Work out the finished part from the listing and answer in its coordinate system (mm). Face numbers are marked on the shaded views. A direction names the side the tool comes from. Give positions to 0.01 mm unless a question says otherwise; leave off trailing zeros. Order: outer loops, then holes, each group sorted by start corner. A loop starts at its lowest first (then second) coordinate and runs counter-clockwise, first axis right, second up. Notation, with made-up numbers: M -35.5,-1 L 10.5,-1 A31 cw 10.5,26 Z; hole C 17,-36.5 d9. An arc over 180 degrees is marked long. One line per item, written item: value.
from build123d import *

# Parameters (mm, degrees)
ESQUISSE1_R             = 24.5
BOSS_EXTRU_1_DEPTH      = 5
ESQUISSE2_R             = 25
BOSS_EXTRU_2_DEPTH      = 2
BOSS_EXTRU_4_START      = 2
ESQUISSE5_R             = 25
BOSS_EXTRU_4_DEPTH      = 2
ESQUISSE4_R             = 1.75
ENL_V_MAT_EXTRU_1_DEPTH = 37.482872694


with BuildPart() as part:
    # Esquisse1 → Boss.-Extru.1 (new body)
    with BuildSketch(Plane.XY):
        Circle(ESQUISSE1_R)
    extrude(amount=BOSS_EXTRU_1_DEPTH)

    # Esquisse2 → Boss.-Extru.2 (add)
    with BuildSketch(Plane(origin=(0, 0, 0), x_dir=(-1, 0, 0), z_dir=(0, 0, -1))):
        Circle(ESQUISSE2_R)
    extrude(amount=BOSS_EXTRU_2_DEPTH)

    # Esquisse5 → Boss.-Extru.4 (add)
    with BuildSketch(Plane.XY.offset(5).offset(BOSS_EXTRU_4_START)):
        with Locations(Location((0, 0, 0), (0, 0, 180))):
            Circle(ESQUISSE5_R)
    extrude(amount=-BOSS_EXTRU_4_DEPTH)

    # Esquisse4 → Enlèv. mat.-Extru.1 (cut, through all)
    with BuildSketch(Plane(origin=(0, 0, -2), x_dir=(-1, 0, 0), z_dir=(0, 0, -1))):
        Circle(ESQUISSE4_R)
    extrude(amount=-ENL_V_MAT_EXTRU_1_DEPTH, mode=Mode.SUBTRACT)


solid = part.part
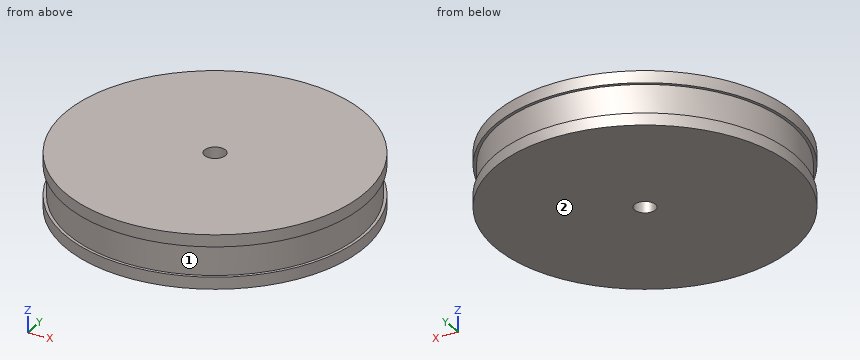
(1) Which of the six approach directions +Z, -Z, +X, -X, +Y, -Y give full straight-line access (tool end or side, diameter ignored) to the marked faces 1 and 2?
Findings:
face 1: none
face 2: -Z, +X, -X, +Y, -Y
(2) Section D-D, the plane y = 18.5 is taken. Give the vertices of the cut face in (x, z).
Findings:
outline: M -16.82,-2 L 16.82,-2 L 16.82,0 L 16.06,0 L 16.06,5 L 16.82,5 L 16.82,7 L -16.82,7 L -16.82,5 L -16.06,5 L -16.06,0 L -16.82,0 Z
(3) Section C-C, the plane z = 3.75 is taken. Give the vertices of the cut face in (x, y), then the cut area to 3 significant figures.
Findings:
outline: C 0,0 d49; hole C 0,0 d3.5
area: 1,880 mm^2
(4) Given P1, Ø3, axis at y = 9.5, z = 3, coming from the +X side; P2, Ø2, axis at y = -2.5, z = 2, coming from the +X side; P3, Ø2, axis at y = 1.5, z = -0.5, coming from the +X side (3 decimals); P4, Ø4.5, axis at x = 0, y = 0, coming from the -Z side, each flat-ended and moving along its own axis, determine where each tip first touches the part or whether it passes through.
Findings:
P1: stops at x = 23.16
P2: stops at x = 24.45
P3: stops at x = 24.995
P4: stops at z = -2
(5) Find the intervals of material crossed by probe 1 along Y at (x, z) = (0, 0.25); probe 2 along X at (y, z) = (-15.5, 0.25); probe 3 along Y at (x, z) = (8, 0.75), in increasing order. Write a range as from..to.
Findings:
probe 1: y = -24.5..-1.75, 1.75..24.5
probe 2: x = -18.97..18.97
probe 3: y = -23.16..23.16
(6) Section A-A, the plane y = 0 is taken. Give the vertices of the cut face in (x, z).
Findings:
outline: M -25,-2 L -1.75,-2 L -1.75,7 L -25,7 L -25,5 L -24.5,5 L -24.5,0 L -25,0 Z; M 1.75,-2 L 25,-2 L 25,0 L 24.5,0 L 24.5,5 L 25,5 L 25,7 L 1.75,7 Z
